Check sheet for the drawn part. Datum: minimum x, y, z corner. Units: mm. A direction names the side the tool comes from. Give positions to 0.01 mm unless a question says otherwise; leave off trailing zeros. Loops run counter-clockwise (first coordinate to the right, second up) from the corner with the lowest first, then second, coordinate; pieces in that order, holes last. Notation, with made-up numbers: (63, 13) - (70, 13) arc R25 cw to (70, 30) - close; hole circle Ø9 at (-6.5, 16.5). An arc over 180 degrees is marked (long way). Answer in a Markdown table with one row per item.
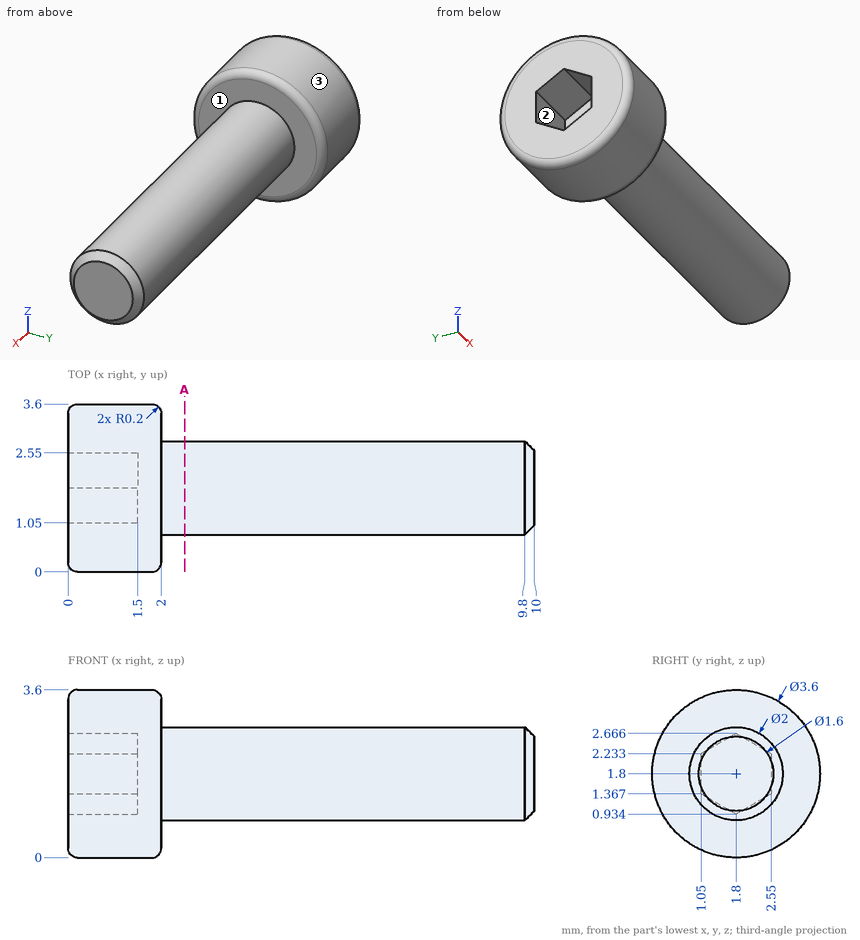
Q1. Sectioned sample at A-A (x = 2.5). Record the cut outline in (y, z).
Completed:
| item | result |
|---|---|
| outline | circle Ø2 at (1.8, 1.8) |
Q2. Tool access check on the marked faces 1, 2 and 3. Record the directions out of +Z, -Z, +X, -X, +Y, -Y that give a thin tool (end or side, any length) a straight path to the whole face; none if there is none.
Completed:
| item | result |
|---|---|
| face 1 | +X |
| face 2 | -X |
| face 3 | +X, -X |
Q3. Thickness scan on line 1 (X direction, y = 1.85, z = 3.25); line 2 (Y direction, x = 1, z = 2.05); line 3 (Z direction, x = 1, y = 1.95). Record the ranges inside material, lowest first.
Completed:
| item | result |
|---|---|
| line 1 | 0 to 2 |
| line 2 | 0.02 to 1.05, 2.55 to 3.58 |
| line 3 | 0.01 to 1.02, 2.58 to 3.59 |
Q4. Go/stop test with a flat-tipped pin: P1, Ø1.5, axis at x = 6.5, z = 3, coming from the -Y side. Record where the tip stops, or that it passes through.
Completed:
| item | result |
|---|---|
| P1 | y = 0.91 |
